from build123d import *

# Parameters (mm, degrees)
SKETCH1_W           = 40
SKETCH1_H           = 7
SKETCH1_R           = 1.5
SKETCH1_W_2         = 82.5
SKETCH1_H_2         = 32
SKETCH1_W_3         = 76.5
SKETCH1_H_3         = 26
BOSS_EXTRUDE1_DEPTH = 2.085
SKETCH2_W           = 5
SKETCH2_H           = 10
BOSS_EXTRUDE2_DEPTH = 3
FILLET1_R           = 2
FILLET2_R           = 2
CUT_EXTRUDE1_DEPTH  = 65.136818612
SKETCH4_W           = 30
SKETCH4_H           = 6.817038716
CUT_EXTRUDE2_DEPTH  = 53.089568977
FILLET3_R           = 5
FILLET4_R           = 2


with BuildPart() as part:
    # Sketch1 → Boss-Extrude1 (new body)
    # profile 1 of 3: a face of its own
    with BuildSketch(Plane(origin=(0, 0, 0), x_dir=(1, 0, 0), z_dir=(0, 1, 0))):
        with Locations((-3.342953498, -16.024946279)):
            Rectangle(SKETCH1_W, SKETCH1_H)
        with Locations(Location((-18.342953498, -14.524946279, 0), (0, 0, 270))):
            Circle(SKETCH1_R, mode=Mode.SUBTRACT)
        with Locations(Location((11.657046502, -14.524946279, 0), (0, 0, 270))):
            Circle(SKETCH1_R, mode=Mode.SUBTRACT)
    # profile 2 of 3: a face of its own
    with BuildSketch(Plane(origin=(0, 0, 0), x_dir=(1, 0, 0), z_dir=(0, 1, 0))):
        with Locations((-3.342953498, 3.475053721)):
            Rectangle(SKETCH1_W_2, SKETCH1_H_2)
        with Locations((-3.342953498, 3.475053721)):
            Rectangle(SKETCH1_W_3, SKETCH1_H_3, mode=Mode.SUBTRACT)
    # profile 3 of 3: a face of its own
    with BuildSketch(Plane(origin=(0, 0, 0), x_dir=(1, 0, 0), z_dir=(0, 1, 0))):
        with Locations((-3.342953498, 22.975053721)):
            Rectangle(SKETCH1_W, SKETCH1_H)
        with Locations(Location((-18.342953498, 21.475053721, 0), (0, 0, 270))):
            Circle(SKETCH1_R, mode=Mode.SUBTRACT)
        with Locations(Location((11.657046502, 21.475053721, 0), (0, 0, 270))):
            Circle(SKETCH1_R, mode=Mode.SUBTRACT)
    extrude(amount=BOSS_EXTRUDE1_DEPTH)

    # Sketch2 → Boss-Extrude2 (add)
    with BuildSketch(Plane.XZ):
        with Locations((-3.342953498, 14.524946279)):
            Rectangle(SKETCH2_W, SKETCH2_H)
        with Locations((-3.342953498, -21.475053721)):
            Rectangle(SKETCH2_W, SKETCH2_H)
    extrude(amount=BOSS_EXTRUDE2_DEPTH)

    # Fillet1
    fillet1_edges = [part.edges().sort_by_distance(p)[0] for p in [
        (-5.842953498, -3, 14.524946279),
        (-0.842953498, -3, 14.524946279),
        (-0.842953498, -3, -21.475053721),
        (-5.842953498, -3, -21.475053721),
    ]]
    fillet(fillet1_edges, radius=FILLET1_R)

    # Fillet2
    fillet2_edges = [part.edges().sort_by_distance(p)[0] for p in [
        (-44.592953498, 1.0425, 12.524946279),
        (-44.592953498, 1.0425, -19.475053721),
        (37.907046502, 1.0425, -19.475053721),
        (37.907046502, 1.0425, 12.524946279),
    ]]
    fillet(fillet2_edges, radius=FILLET2_R)

    # Sketch3 → Cut-Extrude1 (cut, through all)
    with BuildSketch(Plane(origin=(0, 0, -26.475053721), x_dir=(-1, 0, 0), z_dir=(0, 0, -1))):
        with BuildLine():
            Line((5.842953498, -1), (5.842953498, 0))
            Line((5.842953498, 0), (5.642953498, 0))
            Line((5.642953498, 0), (5.642953498, -1))
            ThreePointArc((5.642953498, -1), (5.115745704, -2.272792206), (3.842953498, -2.8))
            Line((3.842953498, -2.8), (2.842953498, -2.8))
            ThreePointArc((2.842953498, -2.8), (1.570161291, -2.272792206), (1.042953498, -1))
            Line((1.042953498, -1), (1.042953498, 0))
            Line((1.042953498, 0), (0.842953498, 0))
            Line((0.842953498, 0), (0.842953498, -1))
            ThreePointArc((0.842953498, -1), (1.428739935, -2.414213562), (2.842953498, -3))
            Line((2.842953498, -3), (3.842953498, -3))
            ThreePointArc((3.842953498, -3), (5.25716706, -2.414213562), (5.842953498, -1))
        make_face()
    extrude(amount=-CUT_EXTRUDE1_DEPTH, mode=Mode.SUBTRACT)

    # Sketch4 → Cut-Extrude2 (cut, through all)
    with BuildSketch(Plane(origin=(0, 2.085, 0), x_dir=(1, 0, 0), z_dir=(0, 1, 0))):
        with BuildLine():
            Line((-5.025587433, 18.475053721), (-3.342953498, 18.475053721))
            Line((-3.342953498, 18.475053721), (-1.660319563, 18.475053721))
            Line((-1.660319563, 18.475053721), (-1.5063675, 18.475053721))
            add(Edge.make_bspline(
                [(7.234880115, 23.808387054), (6.697838422, 22.80689338), (5.54618786, 21.222701251), (3.456402004, 19.887657692), (1.890908212, 19.048171258), (0.265447838, 18.611656881), (-0.841891354, 18.480685845), (-1.5063675, 18.475053721)],
                knots=[0, 0, 0, 0, 0.31493804, 0.524439854, 0.679221784, 0.802825172, 0.985869019, 0.985869019, 0.985869019, 0.985869019], degree=3))
            ThreePointArc((7.234880115, 23.808387054), (9.075057605, 25.756797914), (11.657046502, 26.475053721))
            Line((11.657046502, 26.475053721), (-18.342953498, 26.475053721))
            ThreePointArc((-18.342953498, 26.475053721), (-15.7609646, 25.756797914), (-13.92078711, 23.808387054))
            add(Edge.make_bspline(
                [(-13.92078711, 23.808387054), (-13.383745417, 22.80689338), (-12.232094855, 21.222701251), (-10.142308999, 19.887657692), (-8.576815207, 19.048171258), (-6.951354833, 18.611656881), (-5.844015641, 18.480685845), (-5.179539495, 18.475053721)],
                knots=[0, 0, 0, 0, 0.31493804, 0.524439854, 0.679221784, 0.802825172, 0.985869019, 0.985869019, 0.985869019, 0.985869019], degree=3))
            Line((-5.179539495, 18.475053721), (-5.025587433, 18.475053721))
        make_face()
        with Locations((-3.342953498, 29.883573079)):
            Rectangle(SKETCH4_W, SKETCH4_H)
        with BuildLine():
            ThreePointArc((-13.92078711, -16.858279612), (-15.7609646, -18.806690472), (-18.342953498, -19.524946279))
            Line((-18.342953498, -19.524946279), (11.657046502, -19.524946279))
            ThreePointArc((11.657046502, -19.524946279), (9.075057605, -18.806690472), (7.234880115, -16.858279612))
            add(Edge.make_bspline(
                [(7.234880115, -16.858279612), (6.697838422, -15.856785937), (5.54618786, -14.272593809), (3.456402004, -12.937550249), (1.890908212, -12.098063816), (0.265447838, -11.661549439), (-0.841891354, -11.530578403), (-1.5063675, -11.524946279)],
                knots=[0, 0, 0, 0, 0.31493804, 0.524439854, 0.679221784, 0.802825172, 0.985869019, 0.985869019, 0.985869019, 0.985869019], degree=3))
            Line((-1.5063675, -11.524946279), (-1.660319563, -11.524946279))
            Line((-1.660319563, -11.524946279), (-3.342953498, -11.524946279))
            Line((-3.342953498, -11.524946279), (-5.025587433, -11.524946279))
            Line((-5.025587433, -11.524946279), (-5.179539495, -11.524946279))
            add(Edge.make_bspline(
                [(-13.92078711, -16.858279612), (-13.383745417, -15.856785937), (-12.232094855, -14.272593809), (-10.142308999, -12.937550249), (-8.576815207, -12.098063816), (-6.951354833, -11.661549439), (-5.844015641, -11.530578403), (-5.179539495, -11.524946279)],
                knots=[0, 0, 0, 0, 0.31493804, 0.524439854, 0.679221784, 0.802825172, 0.985869019, 0.985869019, 0.985869019, 0.985869019], degree=3))
        make_face()
        with Locations((-3.342953498, -22.933465637)):
            Rectangle(SKETCH4_W, SKETCH4_H)
    extrude(amount=-CUT_EXTRUDE2_DEPTH, mode=Mode.SUBTRACT)

    # Fillet3
    fillet3_edges = [part.edges().sort_by_distance(p)[0] for p in [
        (16.657046502, 1.0425, -26.475053721),
        (-23.342953498, 1.0425, -26.475053721),
        (-23.342953498, 1.0425, 19.524946279),
        (16.657046502, 1.0425, 19.524946279),
    ]]
    fillet(fillet3_edges, radius=FILLET3_R - 0.0001)  # a hair under: the kernel refuses the full size

    # Fillet4
    fillet4_edges = [part.edges().sort_by_distance(p)[0] for p in [
        (16.657046502, 1.0425, 12.524946279),
        (-23.342953498, 1.0425, 12.524946279),
        (-23.342953498, 1.0425, -19.475053721),
        (16.657046502, 1.0425, -19.475053721),
    ]]
    fillet(fillet4_edges, radius=FILLET4_R)


solid = part.part
Source: CAD feature listing. Evaluate the final solid. Frame: model axes, mm. A direction names the side the tool comes from. Coordinates: 2 decimals unless noted, no trailing zeros. Loops run counter-clockwise (first coordinate to the right, second up) from the corner with the lowest first, then second, coordinate; pieces in that order, holes last. Notation, with made-up numbers: M 37.25,86 L 86.25,86 A9 cw 86.25,103 Z; hole C 50.25,78.25 d4. An arc over 180 degrees is marked long. Answer in a Markdown table with one row per item.
Q1. Section A-A on z = -3. Return the cut outline in (x, y) (3 decimals), plus the area to 3 significant figures.
Answers below:
| item | result |
|---|---|
| outline | M -44.593,0 L -41.593,0 L -41.593,2.085 L -44.593,2.085 Z; M 34.907,0 L 37.907,0 L 37.907,2.085 L 34.907,2.085 Z |
| area | 12.5 mm^2 |
Q2. Draft query along Z for faces 1 (the flat face through (-34, 1, 12.525)), 2 (the flat face through (20, 0, 10)), 3 (the flat face through (-41.593, 1, -3)), 4 (the flat face through (-4, 1, 9.525)). Return one class per face: pulls with the +Z half, pulls with the -Z half, needs draft (parallel to the pull), parting line crosses it, or undercut.
Answers below:
| item | result |
|---|---|
| face 1 | pulls with the +Z half |
| face 2 | needs draft |
| face 3 | undercut |
| face 4 | undercut |
Q3. Set-up query: faces 5 (the flat face through (27, 1, 12.525)), 6 (the flat face through (-4, 1, -16.475)), 7 (the flat face through (-27, 0, 10)), 8 (the flat face through (-3, 0, 11.525)), 9 (the cylindrical face through (-1.6, -2.3, -17.5)). Return all of +Z, -Z, +X, -X, +Y, -Y with unobstructed straight access to the full face (end or side cutting, diameter ignored); none if empty.
Answers below:
| item | result |
|---|---|
| face 5 | +Z, +X, +Y, -Y |
| face 6 | +Y, -Y |
| face 7 | +Z, -Z, -X, -Y |
| face 8 | +Z, +Y, -Y |
| face 9 | +Z, -Z, +X, -Y |
Q4. Ray query, probe 1 along X at (y, z) = (1.2, 7.5); probe 2 along Z at (x, y) = (-5.5, -0.1); probe 3 along Z at (x, y) = (-26, 0.5). Return the intervals inside material, ascending. Write a range as from..to.
Answers below:
| item | result |
|---|---|
| probe 1 | x = -44.59..-41.59, 34.91..37.91 |
| probe 2 | z = -18.48..-16.48, 9.52..11.53 |
| probe 3 | z = -19.48..-16.48, 9.52..12.52 |
Q5. Section B-B on x = -35.5. Return the cut outline in (y, z) (3 decimals).
Answers below:
| item | result |
|---|---|
| outline | M 0,-19.475 L 2.085,-19.475 L 2.085,-16.475 L 0,-16.475 Z; M 0,9.525 L 2.085,9.525 L 2.085,12.525 L 0,12.525 Z |
Q6. Section C-C on y = 1.3. State how many separate pieces and enclosed holes the cut face has, plus the area to 3 significant figures.
Answers below:
| item | result |
|---|---|
| separate pieces | 1 |
| enclosed holes | 5 |
| area | 864 mm^2 |
Q7. First-contact query: pin 1 (1.7 mm diameter, centred on x = -34.5, y = 1.5, fed in from -Z); pin 2 (1.8 mm diameter, centred on x = -4.5, y = 0, fed in from -Z); pin 3 (0.6 mm diameter, centred on x = -30.5, y = 1, fed in from +Z); pin 4 (1.5 mm diameter, centred on x = -26.5, z = -15, fed in from -Y). Flat tips, straight axial feed; report the tip coordinate or a pass-through.
Answers below:
| item | result |
|---|---|
| pin 1 | stops at z = -19.48 |
| pin 2 | stops at z = -18.48 |
| pin 3 | stops at z = 12.52 |
| pin 4 | passes through |
